Build history of the part. All positions in model axes, mm. Face numbers are marked on the shaded views. Give positions to 0.01 mm unless a question says otherwise; leave off trailing zeros. Write each loop counter-clockwise with the first axis right and the second up, starting at its lowest first coordinate (ties: lowest second). Pieces come first, ordered by that corner, then holes.
from build123d import *

# Parameters (mm, degrees)
SKETCH1_R           = 6
SKETCH1_R_2         = 4.1
BOSS_EXTRUDE1_DEPTH = 4
SKETCH5_R           = 2
CUT_EXTRUDE3_DEPTH  = 10


with BuildPart() as part:
    # Sketch1 → Boss-Extrude1 (new body)
    with BuildSketch(Plane.XY):
        with BuildLine():
            Line((-163.238075794, -33.5), (-163.238075794, -90))
            Line((-163.238075794, -90), (-224.321198285, -90))
            ThreePointArc((-224.321198285, -90), (-229.329388299, -92.695755338), (-229.837293325, -98.360655738))
            ThreePointArc((-229.837293325, -98.360655738), (0, -250), (229.837293325, -98.360655738))
            ThreePointArc((229.837293325, -98.360655738), (229.329388299, -92.695755338), (224.321198285, -90))
            Line((224.321198285, -90), (163.238075794, -90))
            Line((163.238075794, -90), (163.238075794, -33.5))
            ThreePointArc((163.238075794, -33.5), (161.480716481, -29.257359313), (157.238075794, -27.5))
            Line((157.238075794, -27.5), (119.238075794, -27.5))
            Line((119.238075794, -27.5), (119.238075794, 27.5))
            Line((119.238075794, 27.5), (157.238075794, 27.5))
            ThreePointArc((157.238075794, 27.5), (161.480716481, 29.257359313), (163.238075794, 33.5))
            Line((163.238075794, 33.5), (163.238075794, 90))
            Line((163.238075794, 90), (224.321198285, 90))
            ThreePointArc((224.321198285, 90), (229.329388299, 92.695755338), (229.837293325, 98.360655738))
            ThreePointArc((229.837293325, 98.360655738), (0, 250), (-229.837293325, 98.360655738))
            ThreePointArc((-229.837293325, 98.360655738), (-229.329388299, 92.695755338), (-224.321198285, 90))
            Line((-224.321198285, 90), (-163.238075794, 90))
            Line((-163.238075794, 90), (-163.238075794, 33.5))
            ThreePointArc((-163.238075794, 33.5), (-161.480716481, 29.257359313), (-157.238075794, 27.5))
            Line((-157.238075794, 27.5), (-119.238075794, 27.5))
            Line((-119.238075794, 27.5), (-119.238075794, -27.5))
            Line((-119.238075794, -27.5), (-157.238075794, -27.5))
            ThreePointArc((-157.238075794, -27.5), (-161.480716481, -29.257359313), (-163.238075794, -33.5))
        make_face()
        with Locations((-141.238075794, 55)):
            Circle(SKETCH1_R, mode=Mode.SUBTRACT)
        with Locations((-141.238075794, -55)):
            Circle(SKETCH1_R, mode=Mode.SUBTRACT)
        with Locations((141.238075794, -55)):
            Circle(SKETCH1_R, mode=Mode.SUBTRACT)
        with Locations((141.238075794, 55)):
            Circle(SKETCH1_R, mode=Mode.SUBTRACT)
        with Locations((0, -202.556165051)):
            Circle(SKETCH1_R_2, mode=Mode.SUBTRACT)
        with Locations((-52.425393218, -195.654231096)):
            Circle(SKETCH1_R_2, mode=Mode.SUBTRACT)
        with Locations((-101.278082525, -175.418784627)):
            Circle(SKETCH1_R_2, mode=Mode.SUBTRACT)
        with Locations((-143.228837878, -143.228837878)):
            Circle(SKETCH1_R_2, mode=Mode.SUBTRACT)
        with Locations((-175.418784627, -101.278082525)):
            Circle(SKETCH1_R_2, mode=Mode.SUBTRACT)
        with Locations((-175.418784627, 101.278082525)):
            Circle(SKETCH1_R_2, mode=Mode.SUBTRACT)
        with Locations((-143.228837878, 143.228837878)):
            Circle(SKETCH1_R_2, mode=Mode.SUBTRACT)
        with Locations((-101.278082525, 175.418784627)):
            Circle(SKETCH1_R_2, mode=Mode.SUBTRACT)
        with Locations((-52.425393218, 195.654231096)):
            Circle(SKETCH1_R_2, mode=Mode.SUBTRACT)
        with Locations((0, 202.556165051)):
            Circle(SKETCH1_R_2, mode=Mode.SUBTRACT)
        with Locations((52.425393218, 195.654231096)):
            Circle(SKETCH1_R_2, mode=Mode.SUBTRACT)
        with Locations((101.278082525, 175.418784627)):
            Circle(SKETCH1_R_2, mode=Mode.SUBTRACT)
        with Locations((143.228837878, 143.228837878)):
            Circle(SKETCH1_R_2, mode=Mode.SUBTRACT)
        with Locations((175.418784627, 101.278082525)):
            Circle(SKETCH1_R_2, mode=Mode.SUBTRACT)
        with Locations((175.418784627, -101.278082525)):
            Circle(SKETCH1_R_2, mode=Mode.SUBTRACT)
        with Locations((143.228837878, -143.228837878)):
            Circle(SKETCH1_R_2, mode=Mode.SUBTRACT)
        with Locations((101.278082525, -175.418784627)):
            Circle(SKETCH1_R_2, mode=Mode.SUBTRACT)
        with Locations((52.425393218, -195.654231096)):
            Circle(SKETCH1_R_2, mode=Mode.SUBTRACT)
    extrude(amount=BOSS_EXTRUDE1_DEPTH)

    # Sketch5 → Cut-Extrude3 (cut)
    with BuildSketch(Plane.XY.offset(4)):
        with Locations((-101.990381057, 146.652521874)):
            Circle(SKETCH5_R)
        with Locations((-76.009618943, 161.652521874)):
            Circle(SKETCH5_R)
        with Locations((-113.990381057, 167.437131564)):
            Circle(SKETCH5_R)
        with Locations((-88.009618943, 182.437131564)):
            Circle(SKETCH5_R)
        with Locations((76.009618943, 161.652521874)):
            Circle(SKETCH5_R)
        with Locations((101.990381057, 146.652521874)):
            Circle(SKETCH5_R)
        with Locations((88.009618943, 182.437131564)):
            Circle(SKETCH5_R)
        with Locations((113.990381057, 167.437131564)):
            Circle(SKETCH5_R)
        with Locations((101.990381057, -146.652521874)):
            Circle(SKETCH5_R)
        with Locations((76.009618943, -161.652521874)):
            Circle(SKETCH5_R)
        with Locations((113.990381057, -167.437131564)):
            Circle(SKETCH5_R)
        with Locations((88.009618943, -182.437131564)):
            Circle(SKETCH5_R)
        with Locations((-76.009618943, -161.652521874)):
            Circle(SKETCH5_R)
        with Locations((-101.990381057, -146.652521874)):
            Circle(SKETCH5_R)
        with Locations((-88.009618943, -182.437131564)):
            Circle(SKETCH5_R)
        with Locations((-113.990381057, -167.437131564)):
            Circle(SKETCH5_R)
    extrude(amount=-CUT_EXTRUDE3_DEPTH, mode=Mode.SUBTRACT)


solid = part.part
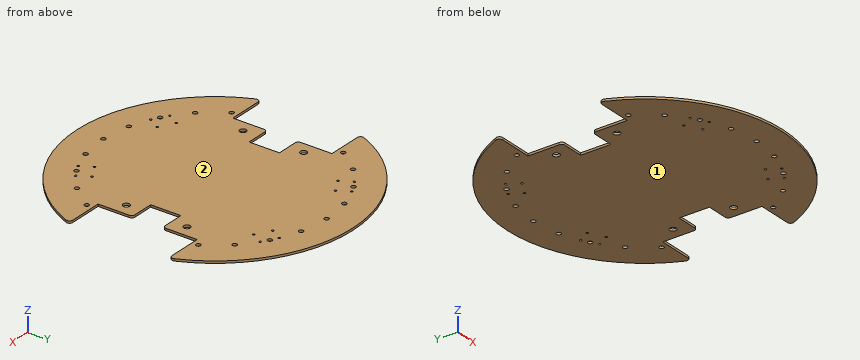
1. Saw through at B-B on x = -197. Give the cut face in (y, z), plus the area to 3 significant figures.
2. Drop flat-ended pins along their axis: pin 1 (6.5 mm diameter, centred on x = 0, y = -202.56, fed in from +Z); pin 2 (1 mm diameter, centred on x = -97, z = 3, fed in from -Y); pin 3 (2 mm diameter, centred on x = 34, z = 3, fed in from -Y); pin 4 (1.2 mm diameter, centred on y = -59, z = 2.5, fed in from +X). Give the stop position or say it passes through.
3. Drill centre lines: line 1 along X through (y, z) = (-58.5, 2.7); line 2 along Y through (x, z) = (53.5, 3.2); line 3 along Y through (x, z) = (-55.5, 1.45). Where is each one in solid material? Low to high.
4. Saw through at D-D on z = 2.9. Count the separate pieces of the cut face and the enclosed holes in it, plus the area to 3 significant figures.
5. Mould opens along Z. For the marked faces 1 and 2 say: pulls with the +Z half, pulls with the -Z half, needs draft (parallel to the pull), parting line crosses it, or undercut.
6. Saw through at C-C on x = 198.5. Give the cut face in (y, z), plus the area to 3 significant figures.
7. Saw through at A-A on y = -55. Give the cut face in (x, z), plus the area to 3 significant figures.
Outcome:
1. outline: (-153.92, 0) - (-90, 0) - (-90, 4) - (-153.92, 4) - close; (90, 0) - (153.92, 0) - (153.92, 4) - (90, 4) - close
1. area: 511 mm2
2. pin 1: passes through
2. pin 2: stops at y = -230.62
2. pin 3: stops at y = -247.81
2. pin 4: stops at x = 163.24
3. line 1: x = -163.24 to -146.11, -136.36 to 136.36, 146.11 to 163.24
3. line 2: y = -244.21 to -199.61, -191.7 to 191.7, 199.61 to 244.21
3. line 3: y = -243.76 to -198.37, -192.94 to 192.94, 198.37 to 243.76
4. separate pieces: 1
4. enclosed holes: 38
4. area: 161,000 mm2
5. face 1: pulls with the -Z half
5. face 2: pulls with the +Z half
6. outline: (-151.98, 0) - (-90, 0) - (-90, 4) - (-151.98, 4) - close; (90, 0) - (151.98, 0) - (151.98, 4) - (90, 4) - close
6. area: 496 mm2
7. outline: (-163.24, 0) - (-147.24, 0) - (-147.24, 4) - (-163.24, 4) - close; (-135.24, 0) - (135.24, 0) - (135.24, 4) - (-135.24, 4) - close; (147.24, 0) - (163.24, 0) - (163.24, 4) - (147.24, 4) - close
7. area: 1,210 mm2
